```python
from build123d import *

# Parameters (mm, degrees)
SKETCH1_R          = 7.62
BASE_EXTRUDE_DEPTH = 177.8
CUT_EXTRUDE1_START = -0.79375
SKETCH2_R          = 7.62
SKETCH2_R_2        = 6.82625
CUT_EXTRUDE1_DEPTH = 0.79375
SKETCH3_R          = 7.62
SKETCH3_R_2        = 6.35
CUT_EXTRUDE2_DEPTH = 15.875


with BuildPart() as part:
    # Sketch1 → Base-Extrude (new body)
    with BuildSketch(Plane(origin=(0, 0, 0), x_dir=(0, 0, -1), z_dir=(1, 0, 0))):
        Circle(SKETCH1_R)
    extrude(amount=BASE_EXTRUDE_DEPTH)

    # Sketch2 → Cut-Extrude1 (cut)
    with BuildSketch(Plane(origin=(165.89375, 0, 0), x_dir=(0, 0, -1), z_dir=(1, 0, 0)).offset(CUT_EXTRUDE1_START)):
        Circle(SKETCH2_R)
        Circle(SKETCH2_R_2, mode=Mode.SUBTRACT)
    extrude(amount=CUT_EXTRUDE1_DEPTH, mode=Mode.SUBTRACT)

    # Sketch3 → Cut-Extrude2 (cut)
    with BuildSketch(Plane.ZY):
        Circle(SKETCH3_R)
        Circle(SKETCH3_R_2, mode=Mode.SUBTRACT)
    extrude(amount=-CUT_EXTRUDE2_DEPTH, mode=Mode.SUBTRACT)


solid = part.part
```
Model file for the job. Use its own axes, mm. A direction names the side the tool comes from. Round coordinates to 2 decimals unless told otherwise and drop trailing zeros. Write each loop counter-clockwise with the first axis right and the second up, starting at its lowest first coordinate (ties: lowest second). Pieces come first, ordered by that corner, then holes. Notation, with made-up numbers: (-3, 55.25) -> (18, 55.25) arc R19 cw to (18, 64.25) -> close; hole circle Ø3 at (8.5, -19). An arc over 180 degrees is marked (long way). Answer as CSV lines item,"result".
1. Slice it at A-A, the plane y = 0. List the corners of the cut face in (x, z) (3 decimals).
Resolved:
outline,"(0, -6.35) -> (15.875, -6.35) -> (15.875, -7.62) -> (165.1, -7.62) -> (165.1, -6.826) -> (165.894, -6.826) -> (165.894, -7.62) -> (177.8, -7.62) -> (177.8, 7.62) -> (165.894, 7.62) -> (165.894, 6.826) -> (165.1, 6.826) -> (165.1, 7.62) -> (15.875, 7.62) -> (15.875, 6.35) -> (0, 6.35) -> close"
2. Tool access for faces 5 (the face through (165.894, -1, 7)), 6 (the face through (7.83, -6.2, -1.38)), 7 (the face through (89.44, -7.44, 1.65)): list every direction of +Z, -Z, +X, -X, +Y, -Y with a clear straight run to the whole face (end or side of a thin tool).
Resolved:
face 5,"none"
face 6,"-X"
face 7,"+X, -X"
3. Drill centre lines: line 1 (Y direction, x = 148.5, z = 0.5); line 2 (Z direction, x = 71, y = 0.25); line 3 (X direction, y = -2.5, z = -7) (3 decimals). Where is each one in solid material? Low to high.
Resolved:
line 1,"-7.6 to 7.6"
line 2,"-7.62 to 7.62"
line 3,"15.875 to 165.1, 165.894 to 177.8"
4. Mould opens along X. For faces 1 (the face through (165.491, 6.768, 0.889)), 2 (the face through (171.76, -7.44, 1.65)), 3 (the face through (165.1, -1, 7)), 4 (the face through (0, 0, 0)) say: +X half, -X half, draft (parallel to the pull), parting line (faces both ways), or undercut.
Resolved:
face 1,"undercut"
face 2,"draft"
face 3,"undercut"
face 4,"-X half"
5. Pin check, flat tips, straight feed: pin 1 Ø5 at (x, z) = (82.5, 5.5) entering from -Y; pin 2 Ø1 at (x, z) = (159, -4.5) entering from -Y; pin 3 Ø4 at (x, z) = (73.5, -4.5) entering from +Y. Stop position of each tip, or through.
Resolved:
pin 1,"y = -7"
pin 2,"y = -6.49"
pin 3,"y = 7.2"
6. Slice it at C-C, the plane x = 91. List the corners of the cut face in (y, z).
Resolved:
outline,"circle Ø15.24 at (0, 0)"
